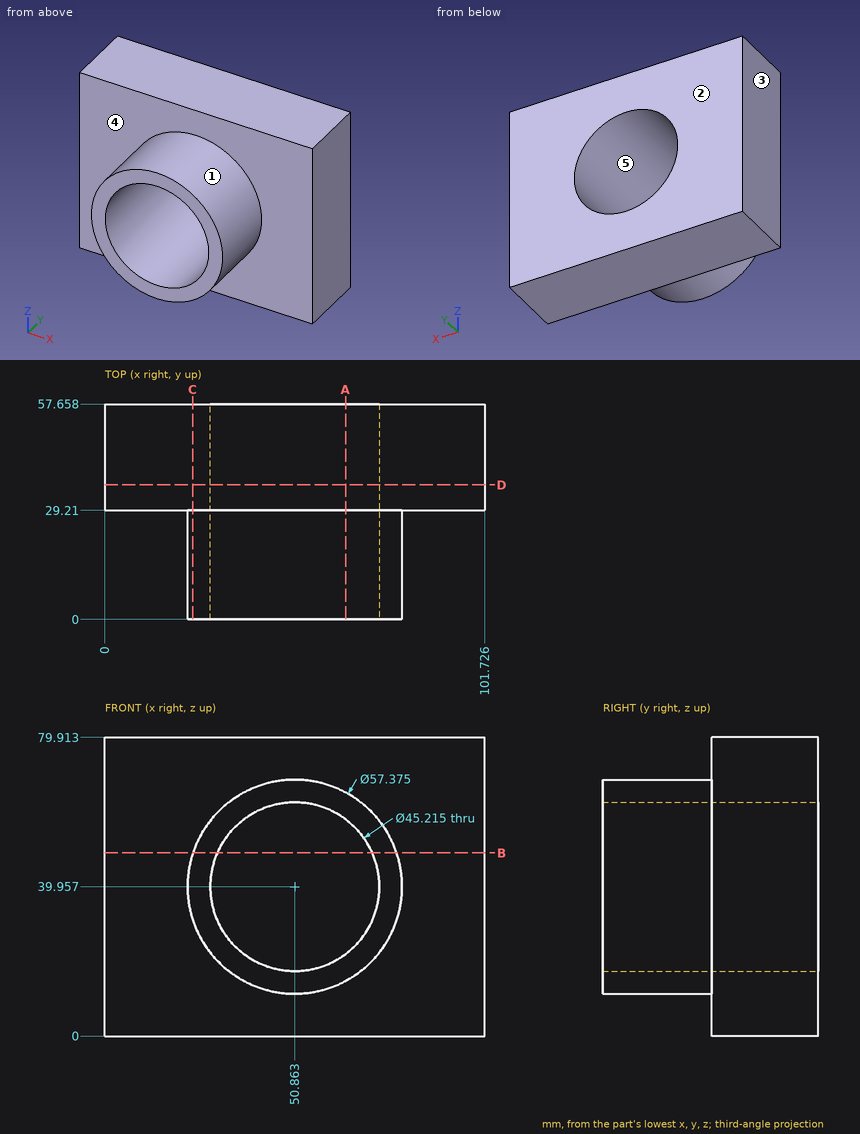
Job drawing, mm, ordinate dimensions from the low corner. One solid piece. A direction names the side the tool comes from. Coordinates: 2 decimals unless noted, no trailing zeros. Order: outer loops, then holes, each group sorted by start corner. A loop starts at its lowest first (then second) coordinate and runs counter-clockwise, first axis right, second up. Notation, with made-up numbers: (-33, 70.5) -> (15, 70.5) arc R19 cw to (15, 75.5) -> close; hole circle Ø5 at (-10, 60). An arc over 180 degrees is marked (long way). Return JSON: item names as keys, results as strings. Group by question number.
Item 1: Saw through at B-B on z = 49. Write the cut outline in (x, y) (1 decimal).
Item 2: Flat gauge pins, fed straight in: P1, Ø10, axis at y = 13.5, z = 45, coming from the -X side (1 decimal); P2, Ø2, axis at y = 18, z = 71, coming from the +X side; P3, Ø6, axis at y = 19.5, z = 27, coming from the +X side; P4, Ø5, axis at x = 58, y = 14, coming from the -Z side. Where does each tip first touch, or does it go through?
Item 3: Saw through at C-C on x = 23.5. Write the cut outline in (y, z).
Item 4: Tool access for the marked faces 1 and 2: list every direction of +Z, -Z, +X, -X, +Y, -Y with a clear straight run to the whole face (end or side of a thin tool).
Item 5: Saw through at D-D on y = 36. Write the cut outline in (x, z) (1 decimal), then the cut area to 3 significant figures.
Item 6: Wall check: line 1 along Y through (x, z) = (19, 44.5); line 2 along X through (y, z) = (27, 45.5) (1 decimal); line 3 along Z through (x, y) = (33, 8.5) (1 decimal). Give the ranges that are in metal, low to high. Write a range as [from, to].
Item 7: Saw through at A-A on x = 64.5. Write the cut outline in (y, z) (1 decimal), then the cut area to 3 significant figures.
Item 8: Pull direction X, two halves, no side cores. Call the marked faces 3, 4 and 5: pulls with the +X half, pulls with the -X half, needs draft (parallel to the pull), parting line crosses it, or undercut.
Values found:
{
 "1": {"outline": "(0, 29.2) -> (23.6, 29.2) -> (23.6, 0) -> (30.1, 0) -> (30.1, 57.7) -> (0, 57.7) -> close; (71.6, 0) -> (78.1, 0) -> (78.1, 29.2) -> (101.7, 29.2) -> (101.7, 57.7) -> (71.6, 57.7) -> close"},
 "2": {"P1": "stops at x = 22.2", "P2": "passes through", "P3": "stops at x = 77.77", "P4": "stops at z = 11.65"},
 "3": {"outline": "(0, 31.34) -> (29.21, 31.34) -> (29.21, 0) -> (57.66, 0) -> (57.66, 79.91) -> (29.21, 79.91) -> (29.21, 48.57) -> (0, 48.57) -> close"},
 "4": {"face 1": "-Y", "face 2": "+Z, -Z, +X, -X, +Y"},
 "5": {"outline": "(0, 0) -> (101.7, 0) -> (101.7, 79.9) -> (0, 79.9) -> close; hole circle Ø45.2 at (50.9, 40)", "area": "6,520 mm2"},
 "6": {"line 1": "y = [29.21, 57.66]", "line 2": "x = [22.7, 28.9], [72.8, 79]", "line 3": "z = [17.5, 26.1], [53.8, 62.4]"},
 "7": {"outline": "(0, 14.7) -> (29.2, 14.7) -> (29.2, 0) -> (57.7, 0) -> (57.7, 21.9) -> (0, 21.9) -> close; (0, 58) -> (57.7, 58) -> (57.7, 79.9) -> (29.2, 79.9) -> (29.2, 65.2) -> (0, 65.2) -> close", "area": "1,670 mm2"},
 "8": {"face 3": "pulls with the -X half", "face 4": "needs draft", "face 5": "undercut"}
}
